Model file for the job. Use its own axes, mm. A direction names the side the tool comes from. Coordinates: 2 decimals unless noted, no trailing zeros. Write each loop counter-clockwise with the first axis right and the second up, starting at its lowest first coordinate (ties: lowest second). Pieces come first, ordered by that corner, then holes.
Q1. Band-saw the part on A-A, the plane y = 0. Write the cut outline in (x, z).
Q2. Pull direction X, two halves, no side cores. Call faces 5 (the flat face through (8, 5, 2)), 6 (the flat face through (0, 0, -3)), 7 (the flat face through (14, 0, 3)): released by +X, released by -X, zero draft, split by the parting line, or undercut.
Q3. Band-saw the part on B-B, the plane z = 0. Write the cut outline in (x, y).
Q4. Band-saw the part on C-C, the plane x = 11. Write the cut outline in (y, z).
Q5. Drill centre lines: probe 1 along X at (y, z) = (5.3, 0); probe 2 along Y at (x, z) = (7, 0); probe 3 along X at (y, z) = (-5, -1.75). Where is each one in solid material? Low to high.
Q6. Band-saw the part on D-D, the plane x = 9. Write the cut outline in (y, z).
Q7. Pin check, flat tips, straight feed: P1, Ø1, axis at x = 6, y = 0.5, coming from the +Z side; P2, Ø1.5, axis at x = 11, y = 0, coming from the -Z side; P3, Ø2, axis at x = 4, z = -2, coming from the +Y side. Stop position of each tip, or through.
Q8. Which spindle directions (+Z, -Z, +X, -X, +Y, -Y) get a long thin tool onto all of the face, cutting with end or side? Do faces 1 (the cylindrical face through (9.75, -0.05, -4.36)), 2 (the cylindrical face through (5, 0, -5)), 3 (the cylindrical face through (9.75, 4.36, -0.05)), 4 (the cylindrical face through (0.256, 3.955, -5.158)). Say none if no direction does.
from build123d import *

# Parameters (mm, degrees)
HOLE_WIZARD_M3_1_REACH   = 22.18
HOLE_WIZARD_M3_1_BORE_R  = 1.25
PATTERN_CIRCULAR_1_COUNT = 2
PATTERN_CIRCULAR_1_ANGLE = 90


with BuildPart() as part:
    # 草图1 → 旋转1 (revolve)
    with BuildSketch(Plane(origin=(0, 0, 0), x_dir=(1, 0, 0), z_dir=(0, 1, 0)), mode=Mode.PRIVATE) as revolve_1_sk:
        Polygon((14, 6.5), (14, 2.5), (0, 2.5), (0, 6.5), (0.504674566, 6.5), (1, 5.642071182), (1, 5), (8, 5), (8, 5.642071182), (8.495325434, 6.5), align=None)
    revolve(revolve_1_sk.sketch.rotate(Axis((-10.793334546, 0, 0), (1, 0, 0)), 180), axis=Axis((-10.793334546, 0, 0), (1, 0, 0)))

    # M3 螺纹孔1 bore → M3 螺纹孔1 (cut, up to next)
    with BuildSketch(Plane(origin=(0, 6.5, 0), x_dir=(1, 0, 0), z_dir=(0, 1, 0)), mode=Mode.PRIVATE) as hole_wizard_m3_1_sk1:
        with Locations((11, 0)):
            Circle(HOLE_WIZARD_M3_1_BORE_R)
    hole_wizard_m3_1_tool1 = extrude(hole_wizard_m3_1_sk1.sketch, amount=-HOLE_WIZARD_M3_1_REACH, mode=Mode.PRIVATE) & part.part
    hole_wizard_m3_1 = hole_wizard_m3_1_tool1.solids().sort_by_distance((11, 6.5, 0))[0]
    add(hole_wizard_m3_1, mode=Mode.SUBTRACT)

    # 阵列(圆周)1: M3 螺纹孔1 ×2 about axis
    pattern_circular_1_axis = Axis((-10.793334546, 0, 0), (-1, 0, 0))
    for i in range(1, PATTERN_CIRCULAR_1_COUNT):
        add(hole_wizard_m3_1.rotate(pattern_circular_1_axis, i * PATTERN_CIRCULAR_1_ANGLE / (PATTERN_CIRCULAR_1_COUNT - 1)), mode=Mode.SUBTRACT)


solid = part.part
Answer sheet:
1. outline: (0, -6.5) - (0.5, -6.5) - (1, -5.64) - (1, -5) - (8, -5) - (8, -5.64) - (8.5, -6.5) - (9.75, -6.5) - (9.75, -2.5) - (0, -2.5) - close; (0, 2.5) - (14, 2.5) - (14, 6.5) - (8.5, 6.5) - (8, 5.64) - (8, 5) - (1, 5) - (1, 5.64) - (0.5, 6.5) - (0, 6.5) - close; (12.25, -6.5) - (14, -6.5) - (14, -2.5) - (12.25, -2.5) - close
2. face 5: undercut
2. face 6: released by -X
2. face 7: released by +X
3. outline: (0, -6.5) - (0.5, -6.5) - (1, -5.64) - (1, -5) - (8, -5) - (8, -5.64) - (8.5, -6.5) - (14, -6.5) - (14, -2.5) - (0, -2.5) - close; (0, 2.5) - (9.75, 2.5) - (9.75, 6.5) - (8.5, 6.5) - (8, 5.64) - (8, 5) - (1, 5) - (1, 5.64) - (0.5, 6.5) - (0, 6.5) - close; (12.25, 2.5) - (14, 2.5) - (14, 6.5) - (12.25, 6.5) - close
4. outline: (-1.25, -6.38) - (-1.25, -2.17) arc R2.5 cw (long way) to (2.17, 1.25) - (6.38, 1.25) arc R6.5 ccw (long way) to start; (1.25, -6.38) arc R6.5 ccw to (6.38, -1.25) - (2.17, -1.25) arc R2.5 cw to (1.25, -2.17) - close
5. probe 1: x = 0 to 1, 8 to 9.75, 12.25 to 14
5. probe 2: y = -5 to -2.5, 2.5 to 5
5. probe 3: x = 0 to 1, 8 to 14
6. outline: circle Ø13 at (0, 0); hole circle Ø5 at (0, 0)
7. P1: stops at z = 5
7. P2: stops at z = 2.38
7. P3: stops at y = 4.9
8. face 1: -Z
8. face 2: none
8. face 3: +Y
8. face 4: +X, -X
